Print and shaded views of the part. All mm, measured from the part's lowest x, y and z. Round coordinates to 2 decimals unless told otherwise and drop trailing zeros. Write each loop counter-clockwise with the first axis right and the second up, starting at its lowest first coordinate (ties: lowest second). Pieces come first, ordered by that corner, then holes. Notation, with made-up numbers: (-27.5, 54) - (22.5, 54) arc R26 ccw to (22.5, 92) - close; hole circle Ø2 at (-38.75, 25.5). An arc over 180 degrees is marked (long way). One line per item, written item: value.
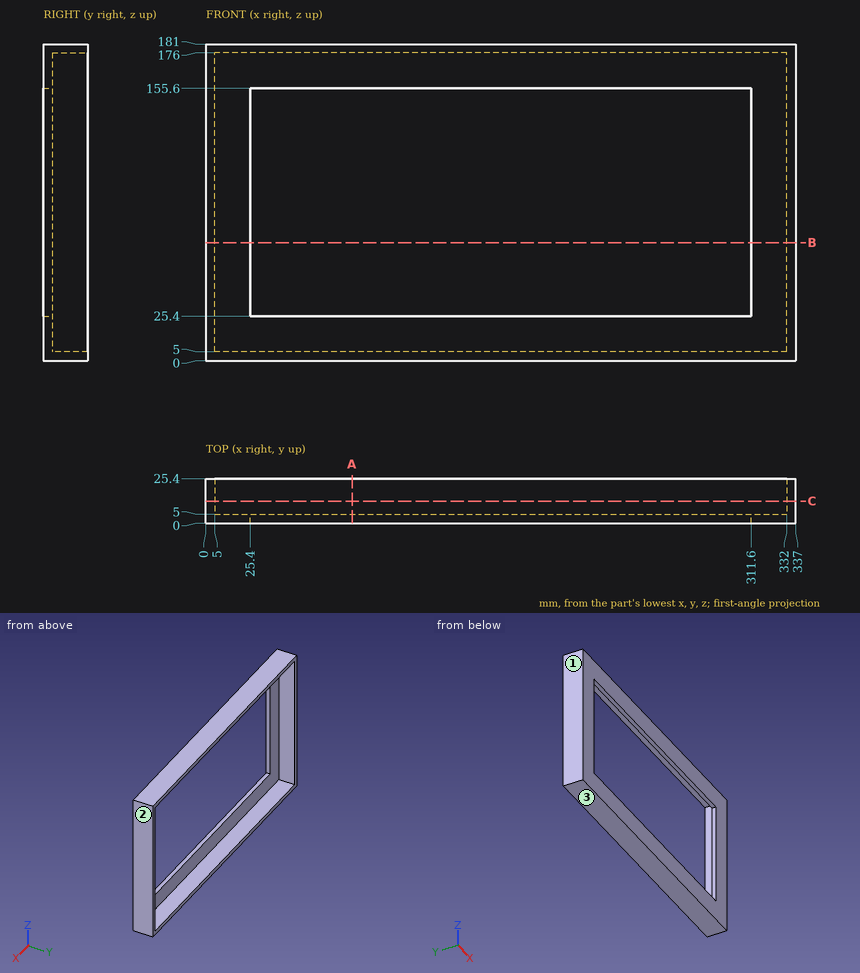
1. Band-saw the part on A-A on x = 83.5. Write the cut outline in (y, z), plus the area to 3 significant figures.
Report:
outline: (0, 0) - (25.4, 0) - (25.4, 5) - (5, 5) - (5, 25.4) - (0, 25.4) - close; (0, 155.6) - (5, 155.6) - (5, 176) - (25.4, 176) - (25.4, 181) - (0, 181) - close
area: 458 mm²
2. Drop flat-ended pins along their axis: pin 1 (10 mm diameter, centred on y = 12, z = 80.5, fed in from -X); pin 2 (6 mm diameter, centred on x = 67.5, z = 157, fed in from +Y). Give the stop position or say it passes through.
Report:
pin 1: x = 0
pin 2: y = 5
3. Mould opens along X. For the marked faces 1, 2 and 3 say: released by +X, released by -X, zero draft, split by the parting line, or undercut.
Report:
face 1: released by -X
face 2: released by +X
face 3: zero draft
4. Band-saw the part on B-B on z = 67.5. Write the cut outline in (x, y).
Report:
outline: (0, 0) - (25.4, 0) - (25.4, 5) - (5, 5) - (5, 25.4) - (0, 25.4) - close; (311.6, 0) - (337, 0) - (337, 25.4) - (332, 25.4) - (332, 5) - (311.6, 5) - close
5. Wall check: probe 1 along Z at (x, y) = (251, 2.75); probe 2 along X at (y, z) = (14, 13.5); probe 3 along Z at (x, y) = (82.5, 12.75). Give the ranges that are in metal, low to high. Write a range as [from, to].
Report:
probe 1: [0, 25.4], [155.6, 181]
probe 2: [0, 5], [332, 337]
probe 3: [0, 5], [176, 181]
6. Band-saw the part on C-C on y = 12.5. Write the cut outline in (x, z), plus the area to 3 significant figures.
Report:
outline: (0, 0) - (337, 0) - (337, 181) - (0, 181) - close; hole (5, 5) - (332, 5) - (332, 176) - (5, 176) - close
area: 5,080 mm²
